from build123d import *

# Parameters (mm, degrees)
ESQUISSE1_W             = 19
ESQUISSE1_H             = 30
BOSS_EXTRU_1_DEPTH      = 1.6
ESQUISSE2_W             = 8
ESQUISSE2_H             = 5.7
BOSS_EXTRU_2_DEPTH      = 2.5
ENL_V_MAT_EXTRU_1_REACH = 37.598
ESQUISSE3_R             = 1.5


with BuildPart() as part:
    # Esquisse1 → Boss.-Extru.1 (new body)
    with BuildSketch(Plane.XY):
        with Locations((9.5, 15)):
            Rectangle(ESQUISSE1_W, ESQUISSE1_H)
    extrude(amount=BOSS_EXTRU_1_DEPTH)

    # Esquisse2 → Boss.-Extru.2 (add)
    with BuildSketch(Plane.XY.offset(1.6)):
        with Locations((9.5, 1.35)):
            Rectangle(ESQUISSE2_W, ESQUISSE2_H)
    extrude(amount=BOSS_EXTRU_2_DEPTH)

    # Esquisse3 → Enlèv. mat.-Extru.1 (cut, up to next)
    with BuildSketch(Plane.XY.offset(1.6), mode=Mode.PRIVATE) as enl_v_mat_extru_1_sk1:
        with Locations((16.4, 3)):
            Circle(ESQUISSE3_R)
    enl_v_mat_extru_1_tool1 = extrude(enl_v_mat_extru_1_sk1.sketch, amount=-ENL_V_MAT_EXTRU_1_REACH, mode=Mode.PRIVATE) & part.part
    # Esquisse3 → Enlèv. mat.-Extru.1 (cut, up to next)
    with BuildSketch(Plane.XY.offset(1.6), mode=Mode.PRIVATE) as enl_v_mat_extru_1_sk2:
        with Locations(Location((2.6, 3, 0), (0, 0, 180))):
            Circle(ESQUISSE3_R)
    enl_v_mat_extru_1_tool2 = extrude(enl_v_mat_extru_1_sk2.sketch, amount=-ENL_V_MAT_EXTRU_1_REACH, mode=Mode.PRIVATE) & part.part
    add(enl_v_mat_extru_1_tool1.solids().sort_by_distance((16.4, 3, 1.6))[0], mode=Mode.SUBTRACT)
    add(enl_v_mat_extru_1_tool2.solids().sort_by_distance((2.6, 3, 1.6))[0], mode=Mode.SUBTRACT)


solid = part.part
The listing builds one solid part. Answer for the finished solid, in the listing's coordinates (mm). A direction names the side the tool comes from. Give positions to 0.01 mm unless a question says otherwise; leave off trailing zeros. Order: outer loops, then holes, each group sorted by start corner. A loop starts at its lowest first (then second) coordinate and runs counter-clockwise, first axis right, second up. Notation, with made-up numbers: (4, 26) - (53, 26) arc R28 cw to (53, 54) - close; hole circle Ø3 at (73.25, 19.25). An arc over 180 degrees is marked (long way). Answer as CSV lines item,"result".
Q1. Which of the six approach directions +Z, -Z, +X, -X, +Y, -Y give full straight-line access (tool end or side, diameter ignored) to faces 4 (the face through (13.5, 1, 3)), 5 (the face through (9, -1, 1.6)), 6 (the face through (9, 4.2, 3))?
Answer key:
face 4,"+Z, +X, +Y, -Y"
face 5,"-Z, +X, -X, -Y"
face 6,"+Z, +X, -X, +Y"
Q2. Each of these flat-tipped pins is pushed along its axis until it touches: pin 1 Ø0.8 at (x, y) = (10, -0.5) entering from -Z; pin 2 Ø0.7 at (y, z) = (2.5, 3) entering from +X; pin 3 Ø0.7 at (y, z) = (0.5, 3.5) entering from -X. Where does it stop, or does it pass through?
Answer key:
pin 1,"stops at z = 1.6"
pin 2,"stops at x = 13.5"
pin 3,"stops at x = 5.5"
Q3. A cutting plane is placed at B-B, the plane x = 2.6. Determine the outline of the cut face in (y, z).
Answer key:
outline,"(0, 0) - (1.5, 0) - (1.5, 1.6) - (0, 1.6) - close; (4.5, 0) - (30, 0) - (30, 1.6) - (4.5, 1.6) - close"
Q4. Straight lines are drawn through the part: L1, parallel to Y at x = 2.6, z = 0.75; L2, parallel to Y at x = 7.5, z = 3.65; L3, parallel to Z at x = 9.25, y = 7. For each, find the intervals that lie inside material, in ascending order.
Answer key:
L1,"y = 0 to 1.5, 4.5 to 30"
L2,"y = -1.5 to 4.2"
L3,"z = 0 to 1.6"
Q5. A cutting plane is placed at D-D, the plane x = 6.5. Determine the outline of the cut face in (y, z), and give its area (4 significant figures).
Answer key:
outline,"(-1.5, 1.6) - (0, 1.6) - (0, 0) - (30, 0) - (30, 1.6) - (4.2, 1.6) - (4.2, 4.1) - (-1.5, 4.1) - close"
area,"62.25 mm^2"
Q6. Determine the mould class of faces 1 (the face through (17.786, 2.425, 0.811)), 2 (the face through (5.5, 1, 3)), 3 (the face through (9, 0, 1)) for opening direction Y: pulls with the +Y half, pulls with the -Y half, needs draft (parallel to the pull), parting line crosses it, or undercut.
Answer key:
face 1,"undercut"
face 2,"needs draft"
face 3,"pulls with the -Y half"
Q7. A cutting plane is placed at A-A, the plane y = 3. Determine the outline of the cut face in (x, z), and give its area (3 significant figures).
Answer key:
outline,"(0, 0) - (1.1, 0) - (1.1, 1.6) - (0, 1.6) - close; (4.1, 0) - (14.9, 0) - (14.9, 1.6) - (13.5, 1.6) - (13.5, 4.1) - (5.5, 4.1) - (5.5, 1.6) - (4.1, 1.6) - close; (17.9, 0) - (19, 0) - (19, 1.6) - (17.9, 1.6) - close"
area,"40.8 mm^2"
Q8. A cutting plane is placed at C-C, the plane z = 0.8. Determine the outline of the cut face in (x, y).
Answer key:
outline,"(0, 0) - (19, 0) - (19, 30) - (0, 30) - close; hole circle Ø3 at (2.6, 3); hole circle Ø3 at (16.4, 3)"
